```python
from build123d import *

# Parameters (mm, degrees)
SKETCH1_R            = 5.44942
BOSS_EXTRUDE1_DEPTH  = 4.763
M3_CLEARANCE_HOLE1_D = 3.2


with BuildPart() as part:
    # Sketch1 → Boss-Extrude1 (new body)
    with BuildSketch(Plane.XY):
        with BuildLine():
            ThreePointArc((10.5, 21.439339413), (13.428932188, 28.510407225), (20.5, 31.439339413))
            Line((20.5, 31.439339413), (22.5, 31.439339413))
            ThreePointArc((22.5, 31.439339413), (28.581287214, 40.95144642), (17.395155109, 42.478758572))
            ThreePointArc((17.395155109, 42.478758572), (17.105956053, 42.072123099), (16.807253326, 41.672416728))
            ThreePointArc((16.807253326, 41.672416728), (0, 33.374189215), (-16.807253326, 41.672416728))
            ThreePointArc((-16.807253326, 41.672416728), (-17.105956053, 42.072123099), (-17.395155109, 42.478758572))
            ThreePointArc((-17.395155109, 42.478758572), (-28.581287214, 40.95144642), (-22.5, 31.439339413))
            Line((-22.5, 31.439339413), (-20.5, 31.439339413))
            ThreePointArc((-20.5, 31.439339413), (-13.428932188, 28.510407225), (-10.5, 21.439339413))
            Line((-10.5, 21.439339413), (-10.5, 0))
            ThreePointArc((-10.5, 0), (0, -10.5), (10.5, 0))
            Line((10.5, 0), (10.5, 21.439339413))
        make_face()
        Circle(SKETCH1_R, mode=Mode.SUBTRACT)
    extrude(amount=BOSS_EXTRUDE1_DEPTH)

    # M3 Clearance Hole1 (through all)
    with Locations(Plane.XY.offset(4.763)):
        with Locations((-22.5, 38.195891618), (22.5, 38.195891618)):
            Hole(M3_CLEARANCE_HOLE1_D / 2)


solid = part.part
```
Geometry check sheet. Reference: the model listing, model coordinates, mm. A direction names the side the tool comes from. Round coordinates to 2 decimals unless told otherwise and drop trailing zeros. Order: outer loops, then holes, each group sorted by start corner. A loop starts at its lowest first (then second) coordinate and runs counter-clockwise, first axis right, second up. Notation, with made-up numbers: (37, 51.5) - (82, 51.5) arc R25 cw to (82, 79.5) - close; hole circle Ø4 at (-15, 67). An arc over 180 degrees is marked (long way). Use a Markdown table: item, result. Add a question column.
1) Thickness scan on line 1 along Y through (x, z) = (-22.5, 1.95); line 2 along Y through (x, z) = (0, 1.75); line 3 along X through (y, z) = (12, 2.15). Record the ranges inside material, lowest first.
2) Mould release check, pull along Y, two halves, no side actions. Record for faces 4 (the cylindrical face through (28.658, 40.78, 2.348)), 5 (the cylindrical face through (-13.51, 28.59, 2.35)), 6 (the cylindrical face through (-23.36, 39.545, 2.348)): released by +Y, released by -Y, zero draft, split by the parting line, or undercut.
3) Set-up check for faces 1 (the flat face through (-10.5, 11, 2)), 2 (the flat face through (0, 24, 0)), 3 (the flat face through (21, 31.439, 2)): record each of +Z, -Z, +X, -X, +Y, -Y from which the full face is reachable in a straight line by a thin tool's end or side.
4) Gauge pin test, flat end, axial feed: P1, Ø1, axis at x = 22, z = 1.5, coming from the -Y side. Record the tip position at first contact, or that the pin passes through.
5) Section check A-A (y = 37.5). Record the cut outline in (x, z).
6) Section check B-B (z = 3.15). Record the cut outline in (x, y).
7) Section check C-C (y = 14). Record the cut outline in (x, z).
8) Section check D-D (x = 6.5). Record the cut outline in (y, z).
Established:
| question | item | result |
|---|---|---|
| 1 | line 1 | 31.44 to 36.6, 39.8 to 44.84 |
| 1 | line 2 | -10.5 to -5.45, 5.45 to 33.37 |
| 1 | line 3 | -10.5 to 10.5 |
| 2 | face 4 | split by the parting line |
| 2 | face 5 | released by -Y |
| 2 | face 6 | undercut |
| 3 | face 1 | +Z, -Z, -X, -Y |
| 3 | face 2 | -Z, +X, -X, +Y, -Y |
| 3 | face 3 | +Z, -Z, +X, -Y |
| 4 | P1 | y = 31.44 |
| 5 | outline | (-29.17, 0) - (-23.94, 0) - (-23.94, 4.76) - (-29.17, 4.76) - close; (-21.06, 0) - (-12.56, 0) - (-12.56, 4.76) - (-21.06, 4.76) - close; (12.56, 0) - (21.06, 0) - (21.06, 4.76) - (12.56, 4.76) - close; (23.94, 0) - (29.17, 0) - (29.17, 4.76) - (23.94, 4.76) - close |
| 6 | outline | (-22.5, 31.44) - (-20.5, 31.44) arc R10 cw to (-10.5, 21.44) - (-10.5, 0) arc R10.5 ccw to (10.5, 0) - (10.5, 21.44) arc R10 cw to (20.5, 31.44) - (22.5, 31.44) arc R6.7 ccw (long way) to (17.4, 42.48) arc R21.17 cw to (-17.4, 42.48) arc R6.7 ccw (long way) to start; hole circle Ø3.2 at (-22.5, 38.2); hole circle Ø10.9 at (0, 0); hole circle Ø3.2 at (22.5, 38.2) |
| 7 | outline | (-10.5, 0) - (10.5, 0) - (10.5, 4.76) - (-10.5, 4.76) - close |
| 8 | outline | (-8.25, 0) - (34.4, 0) - (34.4, 4.76) - (-8.25, 4.76) - close |
